Could you check a few things on this model? Use its own coordinates, in mm. Round coordinates to 2 decimals unless told otherwise and drop trailing zeros. Write each loop counter-clockwise with the first axis right and the second up, starting at its lowest first coordinate (ties: lowest second). Pieces come first, ordered by that corner, then holes. Notation, with made-up numbers: M 18.5,38.25 L 42.5,38.25 A27 ccw 42.5,57.25 Z; hole C 49,37 d11. An arc over 180 degrees is marked long. One line per item, written item: value. Start each with the question number.
(1) I'm going to push a flat-ended pin straight in: pin 1 Ø2.5 at (x, z) = (-15, 31) entering from -Y. Where does the tip first touch, or does it pass through?
(2) I want a section at B-B on x = -15. Please give me the cut outline in (y, z), and give its area (3 significant figures).
(3) If I drill on L1, parallel to Z at x = 15, y = 0.3; L2, parallel to Z at x = 15.5, y = 0.6, over which ranges is the centre line in solid material (lowest first)?
(4) I want a section at A-A on z = -31. Please give me the cut outline in (x, y), and give its area (3 significant figures).
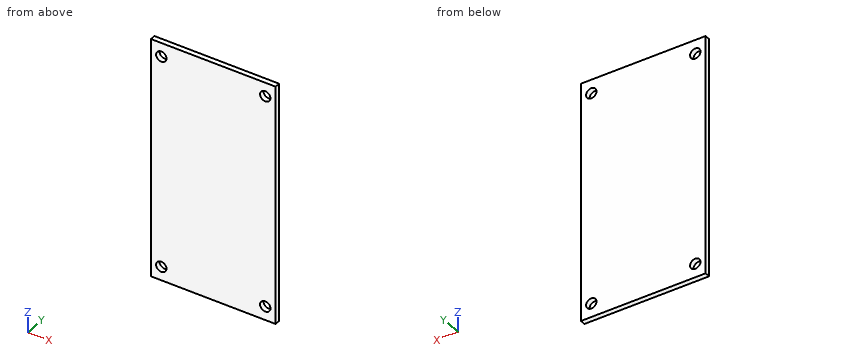
Autodesk Inventor part; units mm, degrees
ref_plane "YZ Plane" through (0, 0, 0) normal (1, 0, 0) x (0, 1, 0)
ref_plane "XZ Plane" through (0, 0, 0) normal (0, 1, 0) x (-1, 0, 0)
ref_plane "XY Plane" through (0, 0, 0) normal (0, 0, 1) x (1, 0, 0)
sketch "Эскиз1" plane through (0, 0, 0) normal (0, 1, 0) x (-1, 0, 0)
  line L0 (-18, -35) -> (18, -35)
  line L1 (18, -35) -> (18, 35)
  line L2 (18, 35) -> (-18, 35)
  line L3 (-18, 35) -> (-18, -35)
  line L4 (-18, -35) -> (18, 35) construction
  line L5 (18, -35) -> (-18, 35) construction
  line L6 (-15, -31) -> (15, -31) construction
  line L7 (15, -31) -> (15, 31) construction
  line L8 (15, 31) -> (-15, 31) construction
  line L9 (-15, 31) -> (-15, -31) construction
  line L10 (-15, -31) -> (15, 31) construction
  line L11 (15, -31) -> (-15, 31) construction
  circle A0 centre (15, 31) radius 1.5
  circle A1 centre (15, -31) radius 1.5
  circle A2 centre (-15, -31) radius 1.5
  circle A3 centre (-15, 31) radius 1.5
  point P0 (0, 0)
  dimension "d0" = 36
  dimension "d1" = 70
  dimension "d2" = 62
  dimension "d3" = 30
  dimension "d4" = 3
  dimension "d5" = 3
  dimension "d6" = 3
  dimension "d7" = 3
extrude "Выдавливание1" add sketch "Эскиз1" along normal blind 1.5
properties part number "DC-DC"
Found:
1. pin 1: passes through
2. outline: M 0,-35 L 1.5,-35 L 1.5,-32.5 L 0,-32.5 Z; M 0,-29.5 L 1.5,-29.5 L 1.5,29.5 L 0,29.5 Z; M 0,32.5 L 1.5,32.5 L 1.5,35 L 0,35 Z
2. area: 96.0 mm²
3. L1: z = -35 to -32.5, -29.5 to 29.5, 32.5 to 35
3. L2: z = -35 to -32.41, -29.59 to 29.59, 32.41 to 35
4. outline: M -18,0 L -16.5,0 L -16.5,1.5 L -18,1.5 Z; M -13.5,0 L 13.5,0 L 13.5,1.5 L -13.5,1.5 Z; M 16.5,0 L 18,0 L 18,1.5 L 16.5,1.5 Z
4. area: 45.0 mm²
